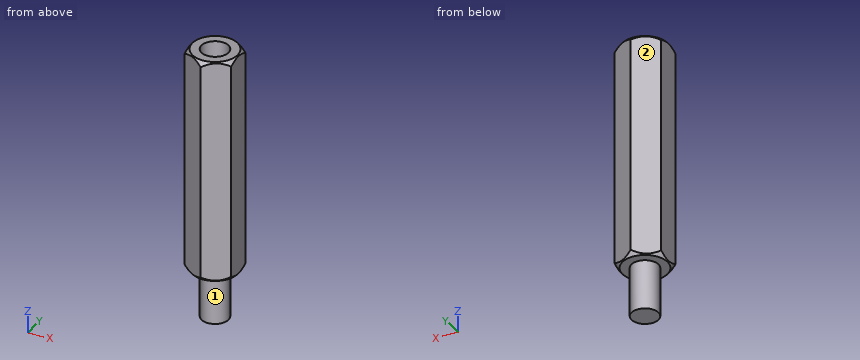
from build123d import *

# Parameters (mm, degrees)
PAD_DEPTH    = 12.5
SKETCH001_R  = 1.5
POCKET_DEPTH = 15
SKETCH002_R  = 1.5
PAD001_DEPTH = 5.5


with BuildPart() as body001:
    # Sketch003 → Revolution (revolve)
    with BuildSketch(Plane.YZ):
        Polygon((2, 13), (5, 13), (5, -13), (2, -13), (3.883364, -11.116636), (3.883364, 11.116636), align=None)
    revolve(axis=Axis((0, 0, 0), (0, 0, 1)))


with BuildPart() as cut:
    # Sketch → Pad (new body, symmetric)
    with BuildSketch(Plane.XY):
        Polygon((2.6, 1.501111), (0, 3.002221), (-2.6, 1.501111), (-2.6, -1.501111), (0, -3.002221), (2.6, -1.501111), align=None)
    extrude(amount=PAD_DEPTH, both=True)

    # Sketch001 (on Face8 of Pad) → Pocket (cut)
    with BuildSketch(Plane.XY.offset(12.5)):
        Circle(SKETCH001_R)
    extrude(amount=-POCKET_DEPTH, mode=Mode.SUBTRACT)

    # Sketch002 (on Face4 of Pocket) → Pad001 (join)
    with BuildSketch(Plane(origin=(0, 0, -12.5), x_dir=(1, 0, 0), z_dir=(0, 0, -1))):
        Circle(SKETCH002_R)
    extrude(amount=PAD001_DEPTH)

    # Cut: cut Body001
    add(body001.part, mode=Mode.SUBTRACT)


solid = cut.part
Part model, mm, in its own coordinate system. Face numbers are marked on the shaded views. A direction names the side the tool comes from. Give positions to 0.01 mm unless a question says otherwise; leave off trailing zeros. Loops run counter-clockwise (first coordinate to the right, second up) from the corner with the lowest first, then second, coordinate; pieces in that order, holes last. Notation, with made-up numbers: M -10,30 L 14,30 A9 cw 14,42 Z; hole C -32.5,33 d9. An arc over 180 degrees is marked long. Put each result on its own line as item: value. Start each with the question number.
1) 3-axis set-ups, long thin cutter, end or side, ignore diameter. For the marked faces 1 and 2: which of +Z, -Z, +X, -X, +Y, -Y reach the whole face in a straight line?
2) Flat gauge pin, fed straight in: pin 1 (1.5 mm diameter, centred on x = 0.5, y = -0.5, fed in from +Z). Where does the tip first touch, or does it go through?
3) Saw through at A-A (z = 0). List the corners of the cut face in (x, y), then the cut area to 3 significant figures.
4) Saw through at C-C (z = -7). List the corners of the cut face in (x, y).
5) Saw through at B-B (y = 0). List the corners of the cut face in (x, z).
6) Probe probe 1 along Z at (x, y) = (0.65, 0.5); probe 2 along Z at (x, y) = (1.1, 2); probe 3 along X at (y, z) = (-0.25, 8.5). List the from-to ranges inside material, lowest first.
Numbers:
1. face 1: -Z
1. face 2: +Z, -Z, -X, +Y
2. pin 1: z = -2.5
3. outline: M -2.6,-1.5 L 0,-3 L 2.6,-1.5 L 2.6,1.5 L 0,3 L -2.6,1.5 Z; hole C 0,0 d3
3. area: 16.3 mm^2
4. outline: M -2.6,-1.5 L 0,-3 L 2.6,-1.5 L 2.6,1.5 L 0,3 L -2.6,1.5 Z
5. outline: M -2.6,-12.4 L -2.5,-12.5 L -1.5,-12.5 L -1.5,-18 L 1.5,-18 L 1.5,-12.5 L 2.5,-12.5 L 2.6,-12.4 L 2.6,12.4 L 2.5,12.5 L 1.5,12.5 L 1.5,-2.5 L -1.5,-2.5 L -1.5,12.5 L -2.5,12.5 L -2.6,12.4 Z
6. probe 1: -18 to -2.5
6. probe 2: -12.5 to 12.5
6. probe 3: -2.6 to -1.48, 1.48 to 2.6
